Here's the drawing with two shaded views (mm, measured from the low corner). I have some questions. Give positions to 0.01 mm unless a question says otherwise; leave off trailing zeros. Write each loop counter-clockwise with the first axis right and the second up, starting at its lowest first coordinate (ties: lowest second). Pieces come first, ordered by that corner, then holes. Notation, with made-up numbers: (49.5, -37.75) -> (53.5, -37.75) arc R29 ccw to (53.5, -6.75) -> close; hole circle Ø7 at (82, 41). An arc over 180 degrees is marked (long way). One line per question, with ' | ' between items.
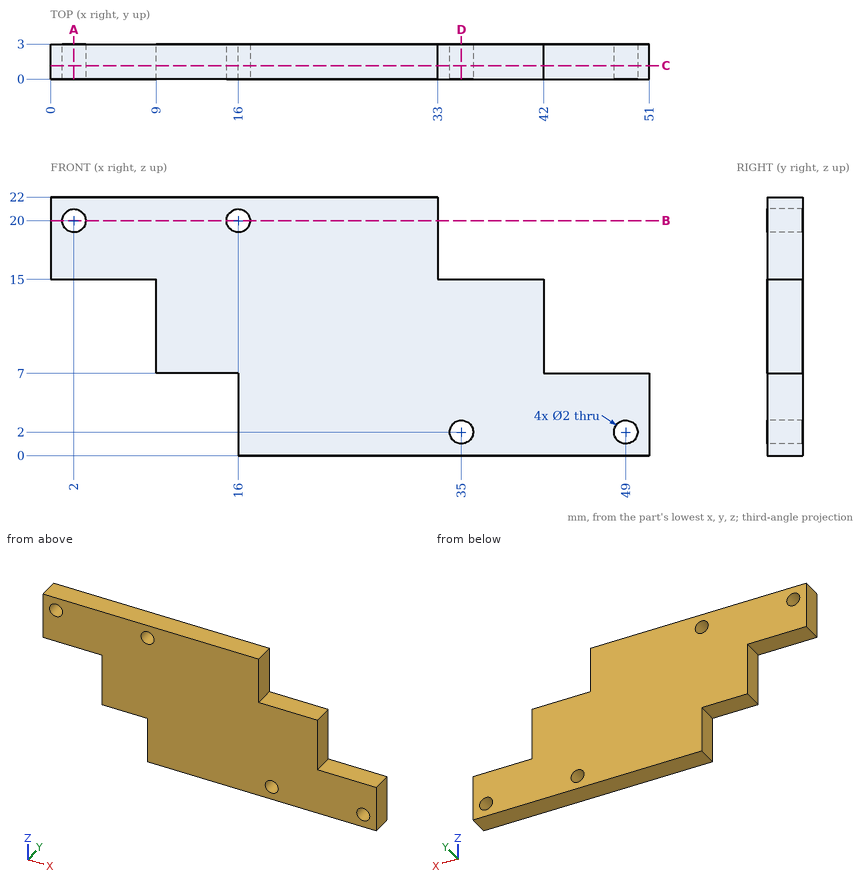
Q1. If I drill on line 1 along Z through (x, y) = (2, 0.65); line 2 along X through (y, z) = (0.25, 1.75); line 3 along Z through (x, y) = (35, 2.1), over which ranges is the centre line in solid material (lowest first)?
Answer below:
line 1: z = 15 to 19, 21 to 22 | line 2: x = 16 to 34.03, 35.97 to 48.03, 49.97 to 51 | line 3: z = 0 to 1, 3 to 15
Q2. Imagine slicing it at A-A on x = 2. Please give me the cut outline in (y, z).
Answer below:
outline: (0, 15) -> (3, 15) -> (3, 19) -> (0, 19) -> close; (0, 21) -> (3, 21) -> (3, 22) -> (0, 22) -> close
Q3. Imagine slicing it at D-D on x = 35. Please give me the cut outline in (y, z), and give its area (3 significant figures).
Answer below:
outline: (0, 0) -> (3, 0) -> (3, 1) -> (0, 1) -> close; (0, 3) -> (3, 3) -> (3, 15) -> (0, 15) -> close | area: 39.0 mm^2
Q4. Imagine slicing it at B-B on z = 20. Please give me the cut outline in (x, y).
Answer below:
outline: (0, 0) -> (1, 0) -> (1, 3) -> (0, 3) -> close; (3, 0) -> (15, 0) -> (15, 3) -> (3, 3) -> close; (17, 0) -> (33, 0) -> (33, 3) -> (17, 3) -> close
Q5. Will these pins go through, and if not, where does the flat tip stop? pin 1 (1.5 mm diameter, centred on x = 12, y = 2, fed in from -Z); pin 2 (0.9 mm diameter, centred on y = 1.5, z = 20, fed in from +X); pin 3 (1.5 mm diameter, centred on y = 1.5, z = 5, fed in from -X); pin 4 (1.2 mm diameter, centred on x = 16, z = 20, fed in from +Y).
Answer below:
pin 1: stops at z = 7 | pin 2: stops at x = 33 | pin 3: stops at x = 16 | pin 4: passes through
Q6. Imagine slicing it at C-C on y = 1.15. Please give me the cut outline in (x, z).
Answer below:
outline: (0, 15) -> (9, 15) -> (9, 7) -> (16, 7) -> (16, 0) -> (51, 0) -> (51, 7) -> (42, 7) -> (42, 15) -> (33, 15) -> (33, 22) -> (0, 22) -> close; hole circle Ø2 at (2, 20); hole circle Ø2 at (16, 20); hole circle Ø2 at (35, 2); hole circle Ø2 at (49, 2)
